The model under review builds one solid part; all positions refer to its coordinate system, in mm. Face numbers are marked on the shaded views. Coordinates: 2 decimals unless noted, no trailing zeros. Order: outer loops, then holes, each group sorted by start corner. A loop starts at its lowest first (then second) coordinate and runs counter-clockwise, first axis right, second up. Notation, with made-up numbers: M 85.25,54.25 L 113.25,54.25 A22 ccw 113.25,91.25 Z; hole C 59,73 d7. An arc over 180 degrees is marked long. One line per item, written item: value.
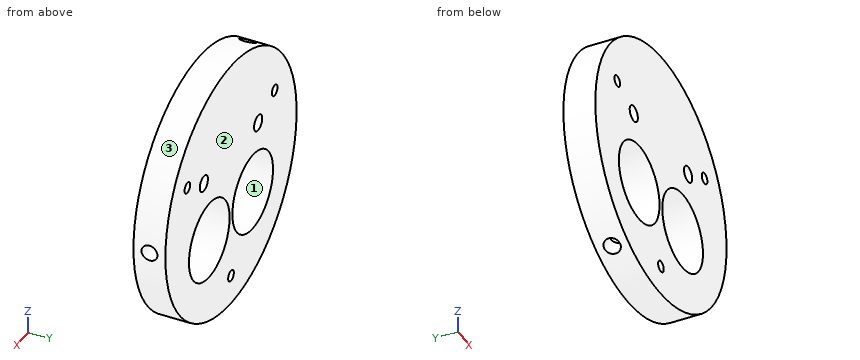
```python
from build123d import *

# Parameters (mm, degrees)
SKETCH1_R               = 38.354
BOSS_EXTRUDE1_DEPTH     = 9.525
SKETCH2_R               = 1.651
SKETCH2_R_2             = 11.8745
CUT_EXTRUDE1_DEPTH      = 10.525
SKETCH4_R               = 2.3749
CUT_EXTRUDE2_DEPTH      = 6.35
CIRPATTERN1_COUNT       = 3
SKETCH5_R               = 2.38125
CUT_EXTRUDE3_DEPTH      = 1.0000001
CUT_EXTRUDE3_DEPTH_BACK = 10.5250001


with BuildPart() as part:
    # Sketch1 → Boss-Extrude1 (new body)
    with BuildSketch(Plane(origin=(0, 0, 0), x_dir=(1, 0, 0), z_dir=(0, 1, 0))):
        Circle(SKETCH1_R)
    extrude(amount=BOSS_EXTRUDE1_DEPTH)

    # Sketch2 → Cut-Extrude1 (cut, through all)
    with BuildSketch(Plane(origin=(0, 9.525, 0), x_dir=(1, 0, 0), z_dir=(0, 1, 0))):
        with Locations((0, 29.464)):
            Circle(SKETCH2_R)
        with Locations((25.516572497, -14.732)):
            Circle(SKETCH2_R)
        with Locations((-25.516572497, -14.732)):
            Circle(SKETCH2_R)
        with Locations((-12.7, 10.16)):
            Circle(SKETCH2_R_2)
        with Locations((12.7, 10.16)):
            Circle(SKETCH2_R_2)
    extrude(amount=-CUT_EXTRUDE1_DEPTH, mode=Mode.SUBTRACT)

    # Sketch4 → Cut-Extrude2 (cut)
    with BuildSketch(Plane(origin=(-19.177, 0, -33.215538337), x_dir=(0, -1, 0), z_dir=(-0.5, 0, -0.866025404))):
        with Locations((-4.7625, 0)):
            Circle(SKETCH4_R)
    cut_extrude2 = extrude(amount=-CUT_EXTRUDE2_DEPTH, mode=Mode.SUBTRACT)

    # CirPattern1: Cut-Extrude2 ×3 about axis
    cirpattern1_axis = Axis((0, 0, 0), (0, 1, 0))
    for i in range(1, CIRPATTERN1_COUNT):
        add(cut_extrude2.rotate(cirpattern1_axis, i * 360 / CIRPATTERN1_COUNT), mode=Mode.SUBTRACT)

    # Sketch5 → Cut-Extrude3 (cut, two sides)
    with BuildSketch(Plane(origin=(0, 9.525, 0), x_dir=(1, 0, 0), z_dir=(0, 1, 0))) as cut_extrude3_sk:
        with Locations((-15.875, -10.16)):
            Circle(SKETCH5_R)
        with Locations((15.875, -10.16)):
            Circle(SKETCH5_R)
    extrude(amount=CUT_EXTRUDE3_DEPTH, mode=Mode.SUBTRACT)
    extrude(cut_extrude3_sk.sketch, amount=-CUT_EXTRUDE3_DEPTH_BACK, mode=Mode.SUBTRACT)


solid = part.part
```
(1) We need section A-A, the plane x = 11. State the section outline as (y, z) points (3 decimals), plus the area to 3 significant figures.
Geometry results:
outline: M 0,-36.743 L 9.525,-36.743 L 9.525,-21.912 L 0,-21.912 Z; M 0,1.592 L 9.525,1.592 L 9.525,36.743 L 0,36.743 Z
area: 476 mm2
(2) We need section B-B, the plane z = 10.16. State the section outline as (x, y) points (3 decimals), plus the area to 3 significant figures.
Geometry results:
outline: M -36.984,0 L -18.256,0 L -18.256,9.525 L -36.984,9.525 Z; M -13.494,0 L 13.494,0 L 13.494,9.525 L -13.494,9.525 Z; M 18.256,0 L 36.984,0 L 36.984,9.525 L 18.256,9.525 Z
area: 614 mm2
(3) Mouldability with a two-part tool opening along X and no side actions: class the marked faces 1, 2 and 3 as +X half, -X half, draft (parallel to the pull), parting line (faces both ways), or undercut.
Geometry results:
face 1: undercut
face 2: draft
face 3: parting line
(4) For L1, parallel to X at y = 3.25, z = -16.5; L2, parallel to X at y = 5, z = -14.5; L3, parallel to Z at x = 0, y = 5.25 (3 decimals), list the stretches that pass through material, from the lowest coordinate up.
Geometry results:
L1: x = -34.62 to -22.74, -2.66 to 2.66, 22.74 to 34.62
L2: x = -35.51 to -23.75, -1.65 to 1.65, 23.75 to 35.51
L3: z = -38.354 to -31.115, -27.813 to 38.354
(5) Insertion check: pin 1 Ø1.5 at (y, z) = (7.5, -22.5) entering from +X; pin 2 Ø4 at (y, z) = (6, 9.5) entering from -X; pin 3 Ø7.5 at (x, z) = (-15.875, 10.16) entering from +Y (3 decimals); pin 4 Ø3 at (x, y) = (10, 4) entering from +Z. Each pin has a flat end and moves straight along its axis. Give the tip position at first contact, or say it passes through.
Geometry results:
pin 1: stops at x = 31.59
pin 2: stops at x = -37.61
pin 3: stops at y = 9.525
pin 4: stops at z = 37.4
(6) We need section C-C, the plane y = 1. State the section outline as (x, z) points (1 decimal), plus the area to 3 significant figures.
Geometry results:
outline: C 0,0 d76.7; hole C -25.5,14.7 d3.3; hole C -12.7,-10.2 d23.7; hole C -15.9,10.2 d4.8; hole C 0,-29.5 d3.3; hole C 12.7,-10.2 d23.7; hole C 15.9,10.2 d4.8; hole C 25.5,14.7 d3.3
area: 3,670 mm2
(7) We need section D-D, the plane z = 0. State the section outline as (x, y) points (3 decimals), plus the area to 3 significant figures.
Geometry results:
outline: M -38.354,0 L -18.846,0 L -18.846,9.525 L -38.354,9.525 Z; M -6.554,0 L 6.554,0 L 6.554,9.525 L -6.554,9.525 Z; M 18.846,0 L 38.354,0 L 38.354,2.388 L 32.004,2.388 L 32.004,7.137 L 38.354,7.137 L 38.354,9.525 L 18.846,9.525 Z
area: 466 mm2
